```python
from build123d import *

# Parameters (mm, degrees)
EXTRUDE_1_DEPTH     = 15
SKETCH_2_W          = 5.6
SKETCH_2_H          = 6
CUT_EXTRUDE_1_DEPTH = 20
SKETCH_3_R          = 1.5
CUT_EXTRUDE_2_DEPTH = 10


with BuildPart() as part:
    # 草图1 → 凸台-拉伸1 (new body, symmetric)
    with BuildSketch(Plane.XY):
        Polygon((0, 0), (18, 0), (18, -30), (0, -30), (0, -42), (3, -42), (3, -33), (21, -33), (21, 3), (3, 3), (3, 12), (0, 12), align=None)
    extrude(amount=EXTRUDE_1_DEPTH, both=True)

    # 草图2 → 切除-拉伸1 (cut)
    with BuildSketch(Plane(origin=(21, 0, 0), x_dir=(0, 0, -1), z_dir=(1, 0, 0))):
        with Locations((-7.2, -5)):
            Rectangle(SKETCH_2_W, SKETCH_2_H)
    cut_extrude_1 = extrude(amount=-CUT_EXTRUDE_1_DEPTH, mode=Mode.SUBTRACT)

    # 镜向1: 切除-拉伸1 across plane
    add(cut_extrude_1.mirror(Plane.XY), mode=Mode.SUBTRACT)

    # 草图3 → 切除-拉伸2 (cut)
    with BuildSketch(Plane(origin=(3, 0, 0), x_dir=(0, 0, -1), z_dir=(1, 0, 0))):
        with Locations((10, 8)):
            Circle(SKETCH_3_R)
        with Locations((-8, 8)):
            Circle(SKETCH_3_R)
    cut_extrude_2 = extrude(amount=-CUT_EXTRUDE_2_DEPTH, mode=Mode.SUBTRACT)

    # 镜向2: 切除-拉伸2 across plane
    add(cut_extrude_2.mirror(Plane(origin=(0, -15, 0), x_dir=(0, 0, 1), z_dir=(0, -1, 0))), mode=Mode.SUBTRACT)


solid = part.part
```
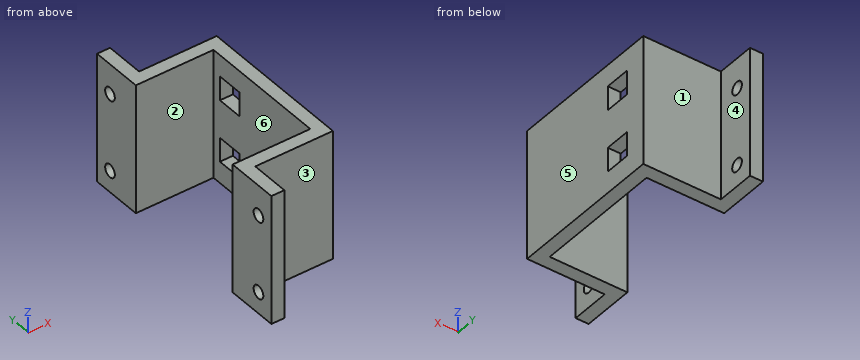
Verification items for the finished model (mm, model axes). Face numbers are marked on the shaded views. A direction names the side the tool comes from. Give positions to 0.01 mm unless a question says otherwise; leave off trailing zeros. Write each loop counter-clockwise with the first axis right and the second up, starting at its lowest first coordinate (ties: lowest second). Pieces come first, ordered by that corner, then holes. Notation, with made-up numbers: M 28,-12 L 79,-12 A25 cw 79,10 Z; hole C 24.25,82.25 d8. An arc over 180 degrees is marked long. One line per question, with ' | ' between items.
1) Set-up check for the marked faces 4, 5 and 6: record each of +Z, -Z, +X, -X, +Y, -Y from which the full face is reachable in a straight line by a thin tool's end or side.
Result:
face 4: +Z, -Z, +X, +Y | face 5: +Z, -Z, +X, +Y, -Y | face 6: +Z, -Z, -X
2) Section check D-D on z = -5. Enter the section's corners in (x, y), plus the area to 3 significant figures.
Result:
outline: M 0,-42 L 3,-42 L 3,-33 L 21,-33 L 21,-8 L 18,-8 L 18,-30 L 0,-30 Z; M 0,0 L 18,0 L 18,-2 L 21,-2 L 21,3 L 3,3 L 3,12 L 0,12 Z | area: 252 mm2
3) Thickness scan on line 1 along Y through (x, z) = (2.45, 8); line 2 along Z through (x, y) = (0.95, -38); line 3 along Y through (x, z) = (16, -5.5). Record the ranges inside material, lowest first. Write a range as [from, to].
Result:
line 1: y = [-42, -39.5], [-36.5, -30], [0, 6.5], [9.5, 12] | line 2: z = [-15, -11.5], [-8.5, 6.5], [9.5, 15] | line 3: y = [-33, -30], [0, 3]
4) Gauge pin test, flat ends, axial feed: pin 1 Ø0.9 at (x, z) = (20, -6.5) entering from +Y; pin 2 Ø2.5 at (y, z) = (8, -10) entering from +X; pin 3 Ø3.5 at (y, z) = (-38, -10) entering from -X; pin 4 Ø5 at (y, z) = (8, 8) entering from +X. Record the tip position at first contact, or that the pin passes through.
Result:
pin 1: stops at y = 3 | pin 2: passes through | pin 3: stops at x = 0 | pin 4: stops at x = 3
5) Mould release check, pull along Y, two halves, no side actions. Record for the marked faces 1, 2 and 3: released by +Y, released by -Y, zero draft, split by the parting line, or undercut.
Result:
face 1: released by +Y | face 2: undercut | face 3: released by -Y
6) Section check C-C on y = -38. Enter the section's corners in (x, z).
Result:
outline: M 0,-15 L 3,-15 L 3,-11.5 L 0,-11.5 Z; M 0,-8.5 L 3,-8.5 L 3,6.5 L 0,6.5 Z; M 0,9.5 L 3,9.5 L 3,15 L 0,15 Z
7) Section check B-B on z = 8. Enter the section's corners in (x, y), plus the area to 3 significant figures.
Result:
outline: M 0,-42 L 3,-42 L 3,-39.5 L 0,-39.5 Z; M 0,-36.5 L 3,-36.5 L 3,-33 L 21,-33 L 21,-8 L 18,-8 L 18,-30 L 0,-30 Z; M 0,0 L 18,0 L 18,-2 L 21,-2 L 21,3 L 3,3 L 3,6.5 L 0,6.5 Z; M 0,9.5 L 3,9.5 L 3,12 L 0,12 Z | area: 234 mm2
8) Section check A-A on x = 15.5. Enter the section's corners in (y, z).
Result:
outline: M -33,-15 L -30,-15 L -30,15 L -33,15 Z; M 0,-15 L 3,-15 L 3,15 L 0,15 Z
